from build123d import *

# Parameters (mm, degrees)
F0_W        = 254
F0_H        = 25.4
F0_R        = 3.175
F1_DEPTH    = 6.35
F2_SIZE     = 0.254
F3_T1_DEPTH = 32.2242991577


# Not quite as in the source:
# - a fillet or chamfer that OpenCascade refuses, or shapes differently, is made with other operations: its cross-section is extruded or revolved along the edge and cut away or added
# - a feature names something its author has since deleted; it is built from what else it names


with BuildPart() as f1:
    # F0 (on Front) → F1 (new body)
    with BuildSketch(Plane.XZ):
        Rectangle(F0_W, F0_H)
        with Locations((-82.55, 0)):
            Circle(F0_R, mode=Mode.SUBTRACT)
        with Locations((-57.15, 0)):
            Circle(F0_R, mode=Mode.SUBTRACT)
        with Locations((-31.75, 0)):
            Circle(F0_R, mode=Mode.SUBTRACT)
        with Locations((-6.35, 0)):
            Circle(F0_R, mode=Mode.SUBTRACT)
        with Locations((19.05, 0)):
            Circle(F0_R, mode=Mode.SUBTRACT)
        with Locations((120.65, 0)):
            Circle(F0_R, mode=Mode.SUBTRACT)
    extrude(amount=F1_DEPTH)

    # F2
    f2_edges = [f1.edges().sort_by_distance(p)[0] for p in [
        (117.475, -6.35, 0),
        (117.475, 0, 0),
        (0, 0, -12.7),
        (127, 0, 0),
        (0, 0, 12.7),
        (-127, 0, 0),
        (-85.725, 0, 0),
        (-60.325, 0, 0),
        (-34.925, 0, 0),
        (-9.525, 0, 0),
        (15.875, 0, 0),
    ]]
    chamfer(f2_edges, length=F2_SIZE)

    # F3: chamfer of 5.08 on 4 edges, made by hand

    # F3_s2 → F3_t1 (cut)
    with BuildSketch(Plane.XZ.offset(-12.8101495789)):
        Polygon((-127, 7.62), (-121.92, 12.7), (-127, 12.7), align=None)
        Polygon((127, 7.62), (121.92, 12.7), (127, 12.7), align=None)
        Polygon((121.92, -12.7), (127, -7.62), (127, -12.7), align=None)
        Polygon((-121.92, -12.7), (-127, -7.62), (-127, -12.7), align=None)
    extrude(amount=F3_T1_DEPTH, mode=Mode.SUBTRACT)


solid = f1.part
Could you check a few things on this model? Use its own coordinates, in mm. Coordinates: 2 decimals unless noted, no trailing zeros. Order: outer loops, then holes, each group sorted by start corner. A loop starts at its lowest first (then second) coordinate and runs counter-clockwise, first axis right, second up.
Q1. Please list where these lines run through material, in increasing order: L1, parallel to Z at x = -6.35, y = -4.5 (3 decimals); L2, parallel to Z at x = -33, y = -3; L3, parallel to X at y = -2.25, z = 10.25.
Q2. Will this pin go through, and if not, where does the flat tip stop? pin 1 (4 mm diameter, centred on x = -82.55, z = 0, fed in from -Y).
Q3. Suppose I cut it at B-B on x = 19.05. Please give me the cut outline in (y, z) (3 decimals), and give its area (3 significant figures).
Q4. Suppose I cut it at A-A on y = -2.5. Please give me the cut outline in (x, z) (3 decimals).
Q5. Thinking about a two-plate mould opening in Z: for faces 1 (the flat face through (124.42, -3.13, -10.2)), 2 (the cylindrical face through (-3.32, -3.26, 0.95)), 3 (the flat face through (-127, -3, 0)), which applies, released by +Z, released by -Z, zero draft, split by the parting line, or undercut?
Answer:
1. L1: z = -12.7 to -3.175, 3.175 to 12.7
1. L2: z = -12.7 to -2.92, 2.92 to 12.7
1. L3: x = -124.37 to 124.37
2. pin 1: passes through
3. outline: (-6.35, -12.7) - (-0.254, -12.7) - (0, -12.446) - (0, -3.429) - (-0.254, -3.175) - (-6.35, -3.175) - close; (-6.35, 3.175) - (-0.254, 3.175) - (0, 3.429) - (0, 12.446) - (-0.254, 12.7) - (-6.35, 12.7) - close
3. area: 121 mm2
4. outline: (-127, -7.62) - (-121.92, -12.7) - (121.92, -12.7) - (127, -7.62) - (127, 7.62) - (121.92, 12.7) - (-121.92, 12.7) - (-127, 7.62) - close; hole circle Ø6.35 at (-82.55, 0); hole circle Ø6.35 at (-57.15, 0); hole circle Ø6.35 at (-31.75, 0); hole circle Ø6.35 at (-6.35, 0); hole circle Ø6.35 at (19.05, 0); hole circle Ø6.35 at (120.65, 0)
5. face 1: released by -Z
5. face 2: undercut
5. face 3: zero draft
